Print and shaded views of the part. All mm, measured from the part's lowest x, y and z. Coordinates: 2 decimals unless noted, no trailing zeros. Order: outer loops, then holes, each group sorted by start corner. A loop starts at its lowest first (then second) coordinate and runs counter-clockwise, first axis right, second up.
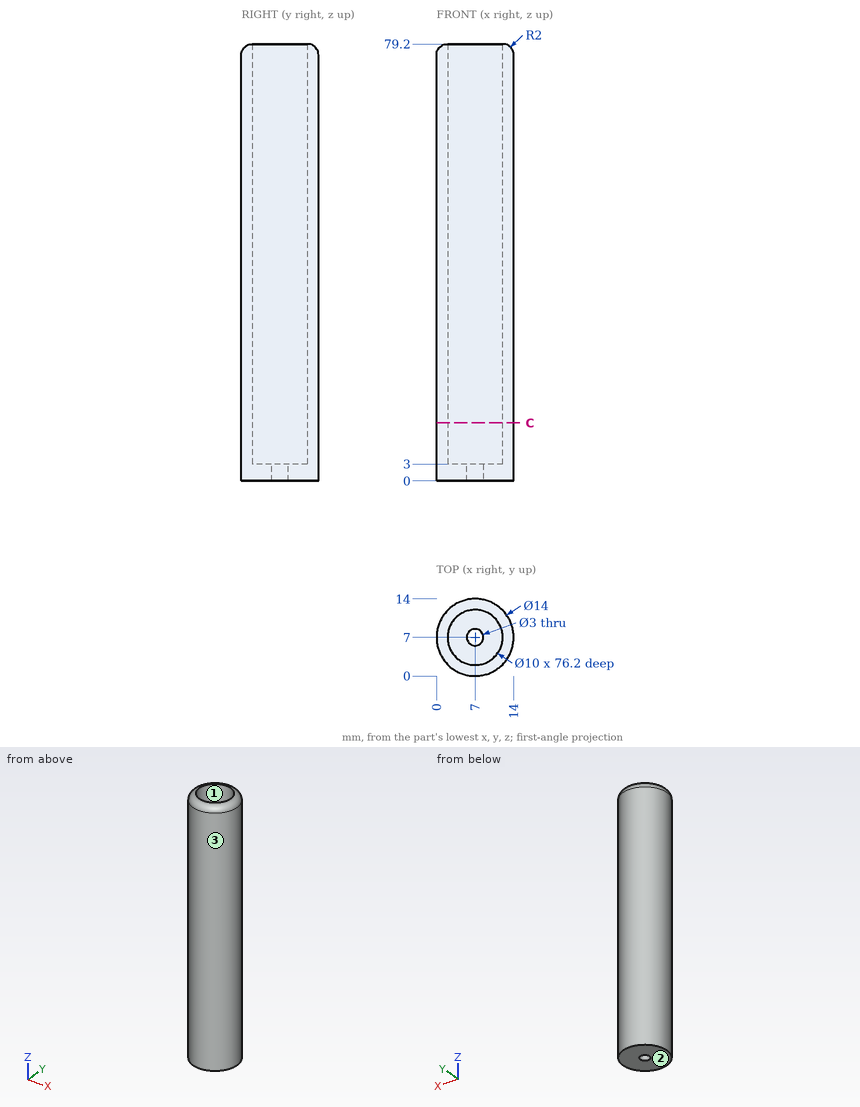
Q1. Mould opens along Y. For the marked faces 1, 2 and 3 say: pulls with the +Y half, pulls with the -Y half, needs draft (parallel to the pull), parting line crosses it, or undercut.
Established:
face 1: undercut
face 2: needs draft
face 3: parting line crosses it
Q2. Probe line 1 (Y direction, x = 7, z = 25); line 2 (Z direction, x = 5.25, y = 7.5); line 3 (Y direction, x = 7, z = 2.15). List the from-to ranges inside material, lowest first.
Established:
line 1: y = 0 to 2, 12 to 14
line 2: z = 0 to 3
line 3: y = 0 to 5.5, 8.5 to 14
Q3. Drop flat-ended pins along their axis: P1, Ø4, axis at x = 11.5, z = 39.5, coming from the -Y side; P2, Ø1, axis at x = 7.5, y = 9, coming from the +Z side. Give the stop position or say it passes through.
Established:
P1: stops at y = 0.46
P2: stops at z = 3
Q4. Cut at C-C, the plane z = 10.5. List the corners of the cut face in (x, y).
Established:
outline: circle Ø14 at (7, 7); hole circle Ø10 at (7, 7)
